Source: CAD feature listing. Evaluate the final solid. Frame: model axes, mm. Face numbers are marked on the shaded views. A direction names the side the tool comes from. Coordinates: 2 decimals unless noted, no trailing zeros. Order: outer loops, then holes, each group sorted by start corner. A loop starts at its lowest first (then second) coordinate and runs counter-clockwise, first axis right, second up.
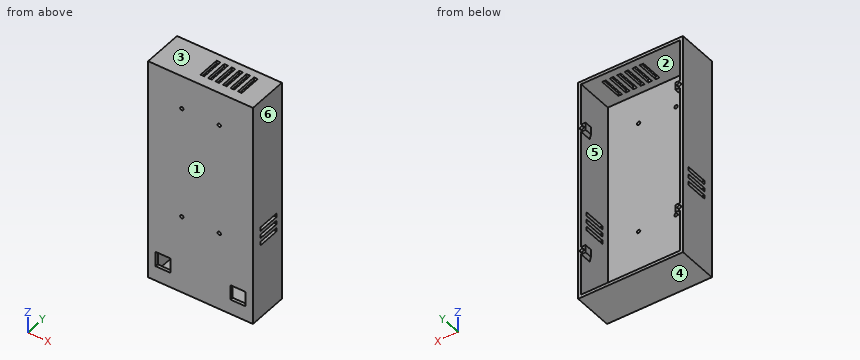
Autodesk Inventor part; units mm, degrees
ref_plane "YZ Plane" through (0, 0, 0) normal (1, 0, 0) x (0, 1, 0)
ref_plane "XZ Plane" through (0, 0, 0) normal (0, 1, 0) x (-1, 0, 0)
ref_plane "XY Plane" through (0, 0, 0) normal (0, 0, 1) x (1, 0, 0)
sketch "Sketch1" plane through (0, 0, 0) normal (0, 1, 0) x (-1, 0, 0)
  line L0 (70, -150) -> (-70, -150)
  line L1 (-70, -150) -> (-70, 150)
  line L2 (-70, 150) -> (70, 150)
  line L3 (70, 150) -> (70, -150)
  line L4 (0, -150) -> (0, 150) construction
  line L5 (70, 0) -> (-70, 0) construction
  point P0 (0, 0)
  point P1 (0, 0)
  dimension "d0" = 140
  dimension "d1" = 300
extrude "Extrusion1" add sketch "Sketch1" along normal blind 4
sketch "Sketch2" plane through (0, 4, 0) normal (0, 1, 0) x (1, 0, 0)
  line L0 (-70, -150) -> (70, -150)
  line L1 (70, -150) -> (70, 150)
  line L2 (-70, -150) -> (70, -150)
  line L3 (70, -150) -> (70, 150)
  line L4 (70, 150) -> (-70, 150)
  line L5 (-70, 150) -> (-70, -150)
  line L6 (-66, -146) -> (66, -146)
  line L7 (66, -146) -> (66, 146)
  line L8 (66, 146) -> (-66, 146)
  line L9 (-66, 146) -> (-66, -146)
  point P0 (0, 0)
  dimension "d4" = 4
  dimension "d5" = 4
  dimension "d6" = 4
  dimension "d7" = 4
extrude "Extrusion2" add sketch "Sketch2" along normal blind 50
sketch "Sketch3" plane through (0, 54, 0) normal (0, 1, 0) x (1, 0, 0)
  line L0 (-70, 150) -> (-70, -150)
  line L1 (-70, -90) -> (-60, -90)
  line L2 (-60, -90) -> (-60, -80)
  line L3 (-60, -80) -> (-70, -80)
  line L4 (-70, -80) -> (-70, -90)
  line L5 (-70, -150) -> (70, -150)
  line L6 (0, -150) -> (0, 150) construction
  line L7 (-70, 150) -> (70, 150) construction
  line L8 (70, -150) -> (70, 150) construction
  line L9 (70, 0) -> (-70, 0) construction
  line L10 (-70, 90) -> (-60, 90)
  line L11 (-60, 90) -> (-60, 80)
  line L12 (-60, 80) -> (-70, 80)
  line L13 (-70, 80) -> (-70, 90)
  line L14 (70, -90) -> (60, -90)
  line L15 (60, -90) -> (60, -80)
  line L16 (60, -80) -> (70, -80)
  line L17 (70, -80) -> (70, -90)
  line L18 (60, 90) -> (60, 80)
  line L19 (70, 90) -> (60, 90)
  line L20 (70, 80) -> (70, 90)
  line L21 (60, 80) -> (70, 80)
  line L22 (65, 80) -> (65, 90) construction
  line L23 (60, 85) -> (70, 85) construction
  circle A0 centre (65, 85) radius 2.5
  circle A1 centre (-65, 85) radius 2.5
  circle A2 centre (65, -85) radius 2.5
  circle A3 centre (-65, -85) radius 2.5
  point P0 (0, 0)
  dimension "d10" = 10
  dimension "d11" = 10
  dimension "d12" = 60
  dimension "d15" = 5
extrude "Extrusion3" add sketch "Sketch3" against normal blind 16 contours L10 L11 L12 L0 | L3 L2 L1 L0 | L14 L15 L16 L17 | L19 L20 L21 L18 | A0 | A1 | A2 | A3
sketch "Sketch4" plane through (0, 54, 0) normal (0, 1, 0) x (1, 0, 0)
  line L0 (70, -150) -> (-70, -150) construction
  line L1 (0, -150) -> (0, 150) construction
  line L2 (-70, 150) -> (70, 150) construction
  line L3 (70, -150) -> (70, 150) construction
  line L4 (70, 0) -> (-70, 0) construction
  line L5 (-70, -150) -> (-70, 150) construction
  line L6 (60, 90) -> (66, 90) construction
  line L7 (60, 90) -> (70, 90) construction
  line L8 (70, 90) -> (70, 80) construction
  line L9 (70, 80) -> (60, 80) construction
  line L10 (60, 80) -> (60, 90) construction
  line L11 (66, 80) -> (60, 80) construction
  line L12 (65, 90) -> (65, 80) construction
  line L13 (60, 80) -> (60, 90) construction
  line L14 (60, 85) -> (70, 85) construction
  circle A0 centre (65, 85) radius 2.5
  circle A1 centre (-65, 85) radius 2.5
  circle A2 centre (65, -85) radius 2.5
  circle A3 centre (-65, -85) radius 2.5
  point P0 (0, 0)
  dimension "d16" = 5
extrude "Extrusion4" cut sketch "Sketch4" against normal blind 6
chamfer "Chamfer1" distance 6 angle 45 4 edges at (60, 38, -85) (60, 38, 85) (-60, 38, -85) (-60, 38, 85)
sketch "Sketch5" plane through (0, 4, 0) normal (0, 1, 0) x (1, 0, 0)
  line L0 (-70, 150) -> (70, 150) construction
  line L1 (0, 150) -> (0, -150) construction
  line L2 (70, -150) -> (-70, -150) construction
  line L3 (60, 110) -> (40, 110)
  line L4 (40, 110) -> (40, 130)
  line L5 (40, 130) -> (60, 130)
  line L6 (60, 130) -> (60, 110)
  line L7 (50, 110) -> (50, 130) construction
  line L8 (60, 120) -> (40, 120) construction
  line L9 (70, -150) -> (70, 150) construction
  line L10 (-60, 110) -> (-40, 110)
  line L11 (-40, 110) -> (-40, 130)
  line L12 (-40, 130) -> (-60, 130)
  line L13 (-60, 130) -> (-60, 110)
  point P0 (0, 0)
  dimension "d22" = 20
  dimension "d23" = 20
  dimension "d24" = 20
  dimension "d26" = 40
extrude "Extrusion5" cut sketch "Sketch5" against normal up to next
sketch "Sketch6" plane through (0, 4, 0) normal (0, 1, 0) x (1, 0, 0)
  line L0 (-57.5, 77.5) -> (57.5, 77.5) construction
  line L1 (57.5, 77.5) -> (57.5, -137.5) construction
  line L2 (57.5, -137.5) -> (-57.5, -137.5) construction
  line L3 (-57.5, -137.5) -> (-57.5, 77.5) construction
  line L4 (-70, 150) -> (70, 150)
  line L5 (0, 150) -> (0, -150) construction
  line L6 (-70, -150) -> (70, -150)
  line L7 (0, 77.5) -> (0, -137.5) construction
  line L8 (-25, 45) -> (25, 45) construction
  line L9 (25, 45) -> (25, -105) construction
  line L10 (25, -105) -> (-25, -105) construction
  line L11 (-25, -105) -> (-25, 45) construction
  line L12 (0, 45) -> (0, -105) construction
  circle A0 centre (-25, 45) radius 2.25
  circle A1 centre (25, 45) radius 2.25
  circle A2 centre (-25, -105) radius 2.25
  circle A3 centre (25, -105) radius 2.25
  line L13 (-66, -146) -> (66, -146)
  point P0 (0, 0)
  dimension "d29" = 115
  dimension "d30" = 215
  dimension "d31" = 50
  dimension "d32" = 150
  dimension "d33" = 32.5
  dimension "d34" = 4.5
  dimension "d35" = 4.5
  dimension "d36" = 4.5
  dimension "d37" = 4.5
  dimension "d38" = 8.5
extrude "Extrusion6" cut sketch "Sketch6" against normal up to next
sketch "Sketch7" plane through (-70, 0, 150) normal (0, 0, 1) x (1, 0, 0)
  line L0 (70, 44) -> (70, 14)
  line L1 (0, 54) -> (140, 54)
  line L2 (140, 0) -> (140, 54)
  line L3 (75, 14) -> (75, 44)
  line L4 (80, 14) -> (80, 44)
  line L5 (85, 14) -> (85, 44)
  line L6 (90, 14) -> (90, 44)
  line L7 (95, 14) -> (95, 44)
  line L8 (100, 14) -> (100, 44)
  line L9 (105, 14) -> (105, 44)
  line L10 (110, 14) -> (110, 44)
  line L11 (115, 14) -> (115, 44)
  line L12 (75, 44) -> (70, 44)
  line L13 (85, 44) -> (80, 44)
  line L14 (95, 44) -> (90, 44)
  line L15 (115, 44) -> (110, 44)
  line L16 (105, 44) -> (100, 44)
  line L17 (70, 14) -> (75, 14)
  line L18 (80, 14) -> (85, 14)
  line L19 (90, 14) -> (95, 14)
  line L20 (100, 14) -> (105, 14)
  line L21 (110, 14) -> (115, 14)
  line L22 (60, 44) -> (60, 14)
  line L23 (65, 14) -> (65, 44)
  line L24 (65, 44) -> (60, 44)
  line L25 (60, 14) -> (65, 14)
  point P0 (70, 0)
  dimension "d42" = 30
  dimension "d45" = 5
  dimension "d47" = 5
  dimension "d48" = 5
  dimension "d49" = 5
  dimension "d50" = 5
  dimension "d51" = 5
  dimension "d52" = 5
  dimension "d53" = 5
  dimension "d54" = 10
  dimension "d55" = 25
  dimension "d56" = 5
  dimension "d60" = 30
  dimension "d61" = 5
  dimension "d62" = 5
extrude "Extrusion7" cut sketch "Sketch7" against normal up to next
sketch "Sketch9" plane through (70, 0, 150) normal (1, 0, 0) x (0, 0, -1)
  line L0 (175, 44) -> (180, 44)
  line L1 (180, 44) -> (180, 14)
  line L2 (180, 14) -> (175, 14)
  line L3 (175, 14) -> (175, 44)
  line L4 (0, 54) -> (300, 54)
  line L5 (185, 44) -> (190, 44)
  line L6 (190, 44) -> (190, 14)
  line L7 (190, 14) -> (185, 14)
  line L8 (185, 14) -> (185, 44)
  line L9 (195, 44) -> (200, 44)
  line L10 (200, 44) -> (200, 14)
  line L11 (200, 14) -> (195, 14)
  line L12 (195, 14) -> (195, 44)
  line L13 (300, 0) -> (300, 54)
  point P0 (150, 0)
  dimension "d63" = 5
  dimension "d64" = 30
  dimension "d65" = 10
  dimension "d68" = 5
  dimension "d69" = 30
  dimension "d70" = 5
  dimension "d71" = 30
  dimension "d72" = 5
  dimension "d73" = 5
  dimension "d74" = 100
extrude "Extrusion8" cut sketch "Sketch9" against normal blind 140
properties part number "power_supply_case"
1. Section query B-B on y = 8. Return loops of the section in (x, z).
Findings:
outline: (-70, -150) - (70, -150) - (70, 150) - (-70, 150) - close; hole (-66, -146) - (66, -146) - (66, 146) - (-66, 146) - close
2. Access query for the marked faces 1 and 2. Directions: +Z, -Z, +X, -X, +Y, -Y. A direction counts if a zero-diameter tool reaches every point of the face in a straight line with its end or side. Return the directions, or none.
Findings:
face 1: +Z, -Z, +X, -X, -Y
face 2: +Y
3. Section query C-C on x = 53. Return loops of the section in (y, z), plus the area to 3 significant figures.
Findings:
outline: (0, -150) - (54, -150) - (54, -146) - (4, -146) - (4, -130) - (0, -130) - close; (0, -110) - (4, -110) - (4, 146) - (54, 146) - (54, 150) - (0, 150) - close
area: 1,520 mm2
4. Section query A-A on z = -119.5. Return loops of the section in (x, y).
Findings:
outline: (-70, 0) - (-60, 0) - (-60, 4) - (-66, 4) - (-66, 54) - (-70, 54) - close; (-40, 0) - (40, 0) - (40, 4) - (-40, 4) - close; (60, 0) - (70, 0) - (70, 54) - (66, 54) - (66, 4) - (60, 4) - close
5. Draft query along Z for the marked faces 3, 4, 5 and 6. Return one class per face: released by +Z, released by -Z, zero draft, split by the parting line, or undercut.
Findings:
face 3: released by +Z
face 4: released by -Z
face 5: undercut
face 6: zero draft
6. Ray query, line 1 (Z direction, x = 25, y = 2.3); line 2 (X direction, y = 50, z = 85); line 3 (Z direction, x = 65, y = 49.2). Return the intervals inside material, ascending.
Findings:
line 1: z = -150 to -47.25, -42.75 to 102.75, 107.25 to 150
line 2: x = -70 to -67.5, -62.5 to -60, 60 to 62.5, 67.5 to 70
line 3: z = -150 to -146, -90 to -87.5, -82.5 to -80, 80 to 82.5, 87.5 to 90, 146 to 150
7. Pin query (flat end, axial travel): P1, Ø4, axis at x = 34.5, z = -7.5, coming from the -Y side. Return the tip coordinate at first contact, or that it passes through.
Findings:
P1: stops at y = 0
8. Section query D-D on z = 58.5. Return loops of the section in (x, y).
Findings:
outline: (-70, 0) - (70, 0) - (70, 54) - (66, 54) - (66, 4) - (-66, 4) - (-66, 54) - (-70, 54) - close
